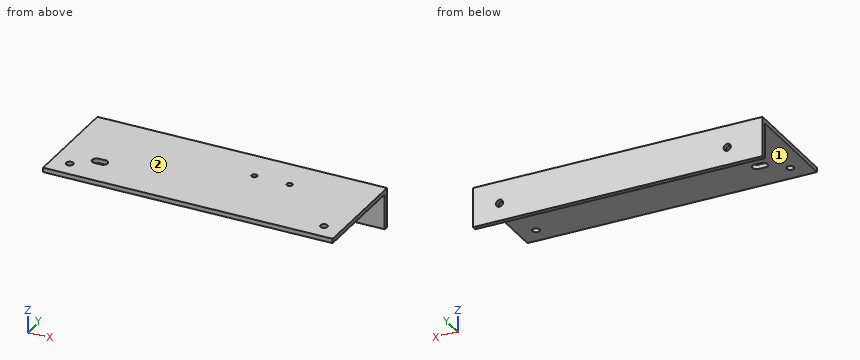
Autodesk Inventor part; units mm, degrees
ref_plane "YZ Plane" through (0, 0, 0) normal (1, 0, 0) x (0, 1, 0)
ref_plane "XZ Plane" through (0, 0, 0) normal (0, 1, 0) x (-1, 0, 0)
ref_plane "XY Plane" through (0, 0, 0) normal (0, 0, 1) x (1, 0, 0)
sketch "Sketch1" plane through (0, 0, 0) normal (1, 0, 0) x (0, 1, 0)
  line L0 (0, 0) -> (76.2, 0)
  line L1 (76.2, 0) -> (76.2, -3.175)
  line L2 (76.2, -3.175) -> (0, -3.175)
  line L3 (0, -3.175) -> (0, 0)
  line L4 (76.2, 0) -> (73.025, 0)
  line L5 (73.025, 0) -> (73.025, -28.575)
  line L6 (73.025, -28.575) -> (76.2, -28.575)
  line L7 (76.2, -28.575) -> (76.2, 0)
  dimension "d0" = 76.2
  dimension "d1" = 3.175
  dimension "d2" = 28.575
extrude "Extrusion1" add sketch "Sketch1" along normal blind 207.9244
sketch "Sketch2" plane through (0, 0, -3.175) normal (0, 0, -1) x (-1, 0, 0)
  line L0 (-207.9244, 0) -> (-207.9244, 73.025)
  line L1 (0, 76.2) -> (-207.9244, 76.2)
  point P0 (0, 0)
  point P1 (-150.4442, 51.9938)
  point P2 (-125.0442, 51.9938)
  dimension "d5" = 57.4802
  dimension "d6" = 82.8802
  dimension "d7" = 24.2062
  dimension "d8" = 24.2062
hole "Hole1" at (150.4442, 51.9938, -3.175) at (125.0442, 51.9938, -3.175) direction (0, 0, 1) diameter 4.0386 end through all
sketch "Sketch5" plane through (0, 76.2, 0) normal (0, 1, 0) x (1, 0, 0)
  line L0 (0, 28.575) -> (207.9244, 28.575)
  line L1 (207.9244, 28.575) -> (207.9244, 0)
  line L2 (0, 28.575) -> (0, 0)
  point P0 (188.8744, 15.875)
  point P1 (25.4, 15.875)
  dimension "d43" = 12.7
  dimension "d44" = 12.7
  dimension "d45" = 19.05
  dimension "d46" = 25.4
sketch "Sketch6" plane through (0, 0, -3.175) normal (0, 0, -1) x (-1, 0, 0)
  line L0 (0, 0) -> (-207.9244, 0)
  line L1 (-207.9244, 0) -> (-207.9244, 73.025)
  line L2 (0, 0) -> (0, 73.025)
  point P0 (-195.2244, 12.7)
  point P1 (-12.7, 12.7)
  dimension "d47" = 12.7
  dimension "d48" = 12.7
  dimension "d49" = 12.7
  dimension "d50" = 12.7
hole "Hole4" at (195.2244, 12.7, -3.175) at (12.7, 12.7, -3.175) direction (0, 0, 1) diameter 5.1054 end through all
hole "Hole3" at (25.4, 76.2, -15.875) at (188.8744, 76.2, -15.875) direction (0, -1, 0) diameter 5.1054 end through all
sketch "Sketch7" plane through (0, 0, 0) normal (0, 0, 1) x (1, 0, 0)
  line L0 (0, 0) -> (207.9244, 0)
  line L1 (207.9244, 76.2) -> (207.9244, 0)
  line L2 (0, 76.2) -> (0, 0)
  point P0 (26.3398, 23.7998)
  dimension "d67" = 23.7998
  dimension "d76" = 26.3398
hole "Hole5" at (26.3398, 23.7998, 0) direction (0, 0, -1) diameter 6.35 end through all
sketch "Sketch8" plane through (0, 0, 0) normal (0, 0, 1) x (1, 0, 0)
  circle A0 centre (26.3398, 23.7998) radius 3.175
  line L0 (26.3398, 23.7998) -> (31.1023, 23.7998) construction
  line L1 (26.3398, 20.6248) -> (31.1023, 20.6248)
  line L2 (31.1023, 26.9748) -> (26.3398, 26.9748)
  arc A1 (26.3398, 26.9748) -> (26.3398, 20.6248) centre (26.3398, 23.7998) ccw
  arc A2 (31.1023, 20.6248) -> (31.1023, 26.9748) centre (31.1023, 23.7998) ccw
  point P0 (0, 0)
  point P1 (28.721, 23.7998)
  dimension "d77" = 4.7625
extrude "Extrusion3" cut sketch "Sketch8" against normal blind 25.4 contours A0 L2 A2 L1
sketch "Sketch3" plane through (0, 0, -3.175) normal (0, 0, -1) x (-1, 0, 0)
  line L0 (-158.5408, 14.5542) -> (38.7343, 14.5542) construction
  line L1 (0, 76.2) -> (-207.9244, 76.2) construction
  line L2 (-161.6607, 44.1198) -> (30.0945, 44.1198) construction
  line L3 (-31.75, 37.7698) -> (-12.7, 37.7698) construction
  line L4 (-31.75, 35.2806) -> (-12.7, 35.2806)
  line L5 (-12.7, 40.259) -> (-31.75, 40.259)
  arc A0 (-31.75, 40.259) -> (-31.75, 35.2806) centre (-31.75, 37.7698) ccw
  arc A1 (-12.7, 35.2806) -> (-12.7, 40.259) centre (-12.7, 37.7698) ccw
  line L6 (-31.75, 25.4) -> (-12.7, 25.4) construction
  line L7 (-31.75, 22.9108) -> (-12.7, 22.9108)
  line L8 (-12.7, 27.8892) -> (-31.75, 27.8892)
  arc A2 (-31.75, 27.8892) -> (-31.75, 22.9108) centre (-31.75, 25.4) ccw
  arc A3 (-12.7, 22.9108) -> (-12.7, 27.8892) centre (-12.7, 25.4) ccw
  line L9 (0, 0) -> (0, 73.025)
  line L10 (-69.85, 37.7698) -> (-50.8, 37.7698) construction
  line L11 (-69.85, 35.2806) -> (-50.8, 35.2806)
  line L12 (-50.8, 40.259) -> (-69.85, 40.259)
  arc A4 (-69.85, 40.259) -> (-69.85, 35.2806) centre (-69.85, 37.7698) ccw
  arc A5 (-50.8, 35.2806) -> (-50.8, 40.259) centre (-50.8, 37.7698) ccw
  point P0 (-22.225, 37.7698)
  point P1 (-22.225, 25.4)
  point P2 (-60.325, 37.7698)
  dimension "d16" = 61.6458
  dimension "d17" = 29.5656
  dimension "d19" = 2.4892
  dimension "d20" = 6.35
  dimension "d29" = 38.1
  dimension "d30" = 6.35
  dimension "d31" = 19.05
  dimension "d32" = 31.75
  dimension "d33" = 31.75
  dimension "d65" = 10.8458
sketch "Sketch4" plane through (0, 0, -3.175) normal (0, 0, -1) x (-1, 0, 0)
  line L0 (-12.7, 35.2806) -> (-31.75, 35.2806)
  arc A0 (-12.7, 22.9108) -> (-12.7, 27.8892) centre (-12.7, 25.4) ccw
  line L1 (-12.7, 22.9108) -> (-31.75, 22.9108)
  arc A1 (-31.75, 27.8892) -> (-31.75, 22.9108) centre (-31.75, 25.4) ccw
  line L2 (-31.75, 27.8892) -> (-12.7, 27.8892)
  arc A2 (-12.7, 35.2806) -> (-12.7, 40.259) centre (-12.7, 37.7698) ccw
  line L3 (-12.7, 35.2806) -> (-31.75, 35.2806)
  arc A3 (-31.75, 40.259) -> (-31.75, 35.2806) centre (-31.75, 37.7698) ccw
  line L4 (-31.75, 40.259) -> (-12.7, 40.259)
  arc A4 (-50.8, 35.2806) -> (-50.8, 40.259) centre (-50.8, 37.7698) ccw
  line L5 (-50.8, 35.2806) -> (-69.85, 35.2806)
  arc A5 (-69.85, 40.259) -> (-69.85, 35.2806) centre (-69.85, 37.7698) ccw
  line L6 (-69.85, 40.259) -> (-50.8, 40.259)
  circle A6 centre (-125.0442, 51.9938) radius 2.0193
  circle A7 centre (-99.6442, 51.9938) radius 2.0193
  line L7 (-182.5244, 73.025) -> (0, 73.025)
  line L8 (-182.5244, 0) -> (-182.5244, 73.025)
  line L9 (0, 0) -> (-182.5244, 0)
  line L10 (0, 0) -> (0, 73.025)
  point P0 (0, 0)
  point P1 (-9.652, 31.5849)
  dimension "d34" = 3.6957
  dimension "d35" = 22.098
  dimension "d66" = 7.3914
equation "\"d30\" = d20"
equation "\"d33\" = d32"
properties part number "CAR_019_TensionerLBracket" material "Aluminum 6061"
Check sheet for the modelled part. Datum: model origin and axes. Units: mm. Face numbers are marked on the shaded views. A direction names the side the tool comes from. Round coordinates to 2 decimals unless told otherwise and drop trailing zeros. Order: outer loops, then holes, each group sorted by start corner. A loop starts at its lowest first (then second) coordinate and runs counter-clockwise, first axis right, second up.
1) Section check B-B (y = 25). Record the boundary of the cut face in (x, z) (3 decimals), and give its area (3 significant figures).
2) Scan lines: line 1 (X direction, y = 12.7, z = -1.55); line 2 (Z direction, x = 89.5, y = 57.5) (3 decimals); line 3 (Y direction, x = 186, z = -20) (3 decimals). Record each from-to range of solid material in increasing order.
3) Section check D-D (y = 52). Record the boundary of the cut face in (x, z) (1 decimal), and give its area (3 significant figures).
4) Section check A-A (y = 12.7). Record the boundary of the cut face in (x, z) (3 decimals).
5) Go/stop test with flat-tipped pins: pin 1 Ø3 at (x, y) = (12.7, 12.7) entering from -Z; pin 2 Ø8 at (x, y) = (94.5, 56.5) entering from -Z (3 decimals); pin 3 Ø4.5 at (x, y) = (125.04, 51.99) entering from +Z; pin 4 Ø8 at (x, z) = (145, -15.5) entering from -Y (3 decimals). Record where each tip stops, or that it passes through.
6) Section check C-C (x = 63). Record the boundary of the cut face in (y, z) (3 decimals), and give its area (3 significant figures).
7) Tool access check on the marked faces 1 and 2. Record the directions out of +Z, -Z, +X, -X, +Y, -Y that give a thin tool (end or side, any length) a straight path to the whole face; none if there is none.
Result:
1. outline: (0, -3.175) - (23.4, -3.175) - (23.4, 0) - (0, 0) - close; (34.042, -3.175) - (207.924, -3.175) - (207.924, 0) - (34.042, 0) - close
1. area: 626 mm2
2. line 1: x = 0 to 10.15, 15.25 to 192.67, 197.78 to 207.92
2. line 2: z = -3.175 to 0
2. line 3: y = 73.025 to 76.2
3. outline: (0, -3.2) - (123, -3.2) - (123, 0) - (0, 0) - close; (127.1, -3.2) - (148.4, -3.2) - (148.4, 0) - (127.1, 0) - close; (152.5, -3.2) - (207.9, -3.2) - (207.9, 0) - (152.5, 0) - close
3. area: 635 mm2
4. outline: (0, -3.175) - (10.147, -3.175) - (10.147, 0) - (0, 0) - close; (15.253, -3.175) - (192.672, -3.175) - (192.672, 0) - (15.253, 0) - close; (197.777, -3.175) - (207.924, -3.175) - (207.924, 0) - (197.777, 0) - close
5. pin 1: passes through
5. pin 2: stops at z = -3.175
5. pin 3: stops at z = 0
5. pin 4: stops at y = 73.025
6. outline: (0, -3.175) - (73.025, -3.175) - (73.025, -28.575) - (76.2, -28.575) - (76.2, 0) - (0, 0) - close
6. area: 323 mm2
7. face 1: -Z, +X, -X, -Y
7. face 2: +Z, +X, -X, +Y, -Y
